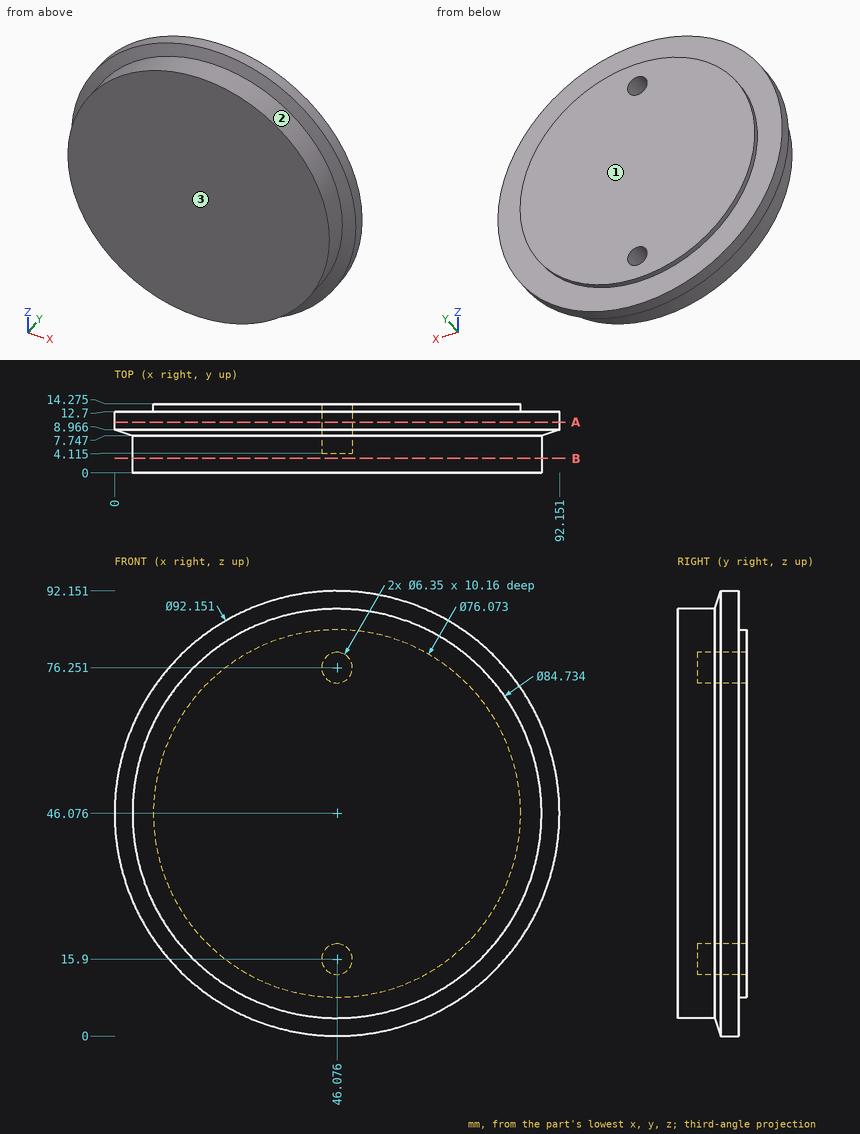
Study the drawing (mm; zero at the part's minimum x, y, z) and answer. Round coordinates to 2 decimals unless told otherwise and drop trailing zeros. Order: outer loops, then holes, each group sorted by start corner. A loop starts at its lowest first (then second) coordinate and runs counter-clockwise, first axis right, second up. Notation, with made-up numbers: (69, 89.5) -> (85, 89.5) arc R21 ccw to (85, 123.5) -> close; hole circle Ø11 at (13.25, -23). An arc over 180 degrees is marked (long way). Write each question's results on one line, items separated by ' | '. Start each with the question number.
Q1. Straight lines are drawn through the part: probe 1 along Y at (x, z) = (79.5, 69); probe 2 along X at (y, z) = (1.5, 46); probe 3 along Y at (x, z) = (44.5, 16) (1 decimal). For each, find the intervals that lie inside material, in ascending order. Write a range as from..to.
Q2. Find section A-A (y = 10.5). Give the number of separate pieces and of enclosed holes in the cut face, then the cut area to 3 significant figures.
Q3. Find section B-B (y = 3). Determine the outline of the cut face in (x, z) (1 decimal), then the cut area to 3 significant figures.
Q4. Each of these flat-tipped pins is pushed along its axis until it touches: pin 1 (5.5 mm diameter, centred on x = 46.08, z = 76.25, fed in from -Y); pin 2 (1.5 mm diameter, centred on y = 5.5, z = 28, fed in from +X); pin 3 (1 mm diameter, centred on x = 45, y = 10.5, fed in from +Z); pin 4 (2 mm diameter, centred on y = 5, z = 18, fed in from -X). Where does it stop, or does it pass through?
Q5. The mould has two halves that part along Y. Classify the marked faces 1, 2 and 3: pulls with the +Y half, pulls with the -Y half, needs draft (parallel to the pull), parting line crosses it, or undercut.
Worked answers:
1) probe 1: y = 0..12.7 | probe 2: x = 3.71..88.44 | probe 3: y = 0..4.1
2) separate pieces: 1 | enclosed holes: 2 | area: 6,610 mm2
3) outline: circle Ø84.7 at (46.1, 46.1) | area: 5,640 mm2
4) pin 1: stops at y = 0 | pin 2: stops at x = 84.74 | pin 3: stops at z = 92.15 | pin 4: stops at x = 13.49
5) face 1: pulls with the +Y half | face 2: needs draft | face 3: pulls with the -Y half
